Job drawing, mm, ordinate dimensions from the low corner. One solid piece. A direction names the side the tool comes from. Give positions to 0.01 mm unless a question says otherwise; leave off trailing zeros. Write each loop counter-clockwise with the first axis right and the second up, starting at its lowest first coordinate (ties: lowest second). Pieces come first, ordered by that corner, then holes. Notation, with made-up numbers: M 73.25,-33 L 95.25,-33 A31 ccw 95.25,4 Z; hole C 55,-27 d9. An arc over 180 degrees is marked long. Answer as CSV lines item,"result". Start each with the question number.
Item 1: Band-saw the part on C-C, the plane z = 1.5. List the corners of the cut face in (x, y), then the cut area to 3 significant figures.
Item 2: Wall check: L1, parallel to Y at x = 2.5, z = 0.8; L2, parallel to Z at x = 4.1, y = 3.5; L3, parallel to X at y = 24, z = 1 (1 decimal). Give the ranges that are in metal, low to high. Write a range as from..to.
Item 3: 3-axis set-ups, long thin cutter, end or side, ignore diameter. For the marked faces 4, 5 and 6: which of +Z, -Z, +X, -X, +Y, -Y reach the whole face in a straight line?
Item 4: Band-saw the part on A-A, the plane y = 2.5. List the corners of the cut face in (x, z).
Item 5: Band-saw the part on B-B, the plane x = 1.8. List the corners of the cut face in (y, z) (1 decimal), then the cut area to 3 significant figures.
Item 6: Two-plate mould, pull along Y, no slides. Class the marked faces 1, 2 and 3: +Y half, -Y half, draft (parallel to the pull), parting line (faces both ways), or undercut.
Item 7: Band-saw the part on D-D, the plane x = 2.95. List the corners of the cut face in (y, z), then the cut area to 3 significant figures.
Item 8: Pin check, flat tips, straight feed: pin 1 (2.5 mm diameter, centred on x = 1.5, z = 3.5, fed in from -Y); pin 2 (2 mm diameter, centred on y = 10.5, z = 6.5, fed in from +X); pin 3 (3 mm diameter, centred on x = 2.5, y = 2.5, fed in from +Z); pin 4 (2 mm diameter, centred on x = 3, z = 6, fed in from +Y). Stop position of each tip, or through.
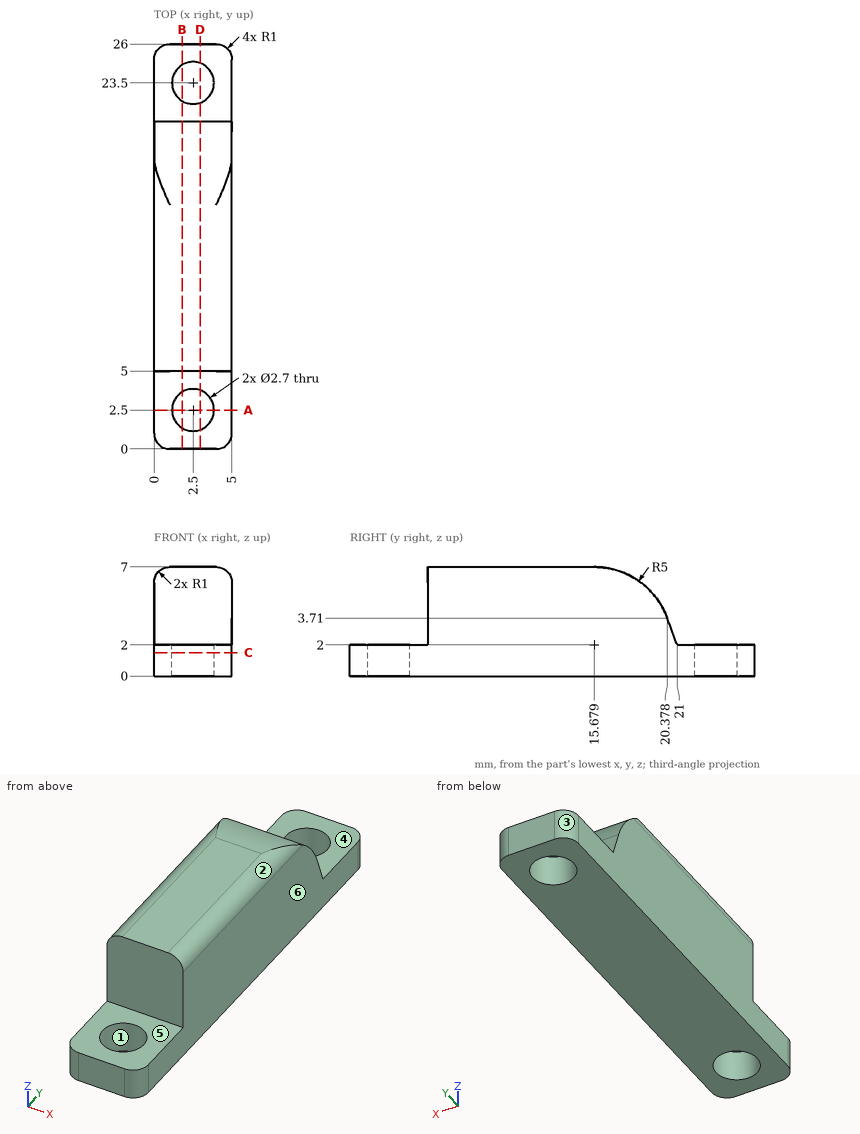
Output:
1,outline,"M 0,1 A1 ccw 1,0 L 4,0 A1 ccw 5,1 L 5,25 A1 ccw 4,26 L 1,26 A1 ccw 0,25 Z; hole C 2.5,2.5 d2.7; hole C 2.5,23.5 d2.7"
1,area,"118 mm²"
2,L1,"0..1.15, 3.85..22.15, 24.85..26"
2,L2,"0..2"
2,L3,"0..1.2, 3.8..5"
3,face 4,"+Z, +X, -X, +Y"
3,face 5,"+Z, +X, -X, -Y"
3,face 6,"+Z, -Z, +X, +Y, -Y"
4,outline,"M 0,0 L 1.15,0 L 1.15,2 L 0,2 Z; M 3.85,0 L 5,0 L 5,2 L 3.85,2 Z"
5,outline,"M 0,0 L 1.3,0 L 1.3,2 L 0,2 Z; M 3.7,0 L 22.3,0 L 22.3,2 L 21,2 L 20.4,3.7 A5 ccw 15.7,7 L 5,7 L 5,2 L 3.7,2 Z; M 24.7,0 L 26,0 L 26,2 L 24.7,2 Z"
5,area,"116 mm²"
6,face 1,"undercut"
6,face 2,"draft"
6,face 3,"+Y half"
7,outline,"M 0,0 L 1.23,0 L 1.23,2 L 0,2 Z; M 3.77,0 L 22.23,0 L 22.23,2 L 21,2 L 20.38,3.71 A5 ccw 15.68,7 L 5,7 L 5,2 L 3.77,2 Z; M 24.77,0 L 26,0 L 26,2 L 24.77,2 Z"
7,area,"115 mm²"
8,pin 1,"y = 5"
8,pin 2,"x = 5"
8,pin 3,"z = 2"
8,pin 4,"y = 19.68"
